Could you check a few things on this model? Use its own coordinates, in mm. Round coordinates to 2 decimals unless told otherwise and drop trailing zeros. Order: outer loops, then holes, each group sorted by start corner. A loop starts at its lowest first (then second) coordinate and runs counter-clockwise, first axis right, second up.
```python
from build123d import *

# Parameters (mm, degrees)
ESBO_O1_R                = 3
RESSALTO_EXTRUS_O1_DEPTH = 36
CHANFRO1_SIZE            = 0.25
ESBO_O2_R                = 2
CORTE_EXTRUS_O1_DEPTH    = 16


with BuildPart() as part:
    # Esboço1 → Ressalto-extrusão1 (new, symmetric)
    with BuildSketch(Plane.XY):
        Circle(ESBO_O1_R)
    extrude(amount=RESSALTO_EXTRUS_O1_DEPTH, both=True)

    # Chanfro1
    chanfro1_edges = [part.edges().sort_by_distance(p)[0] for p in [
        (-3, 0, -36),
        (-3, 0, 36),
    ]]
    chamfer(chanfro1_edges, length=CHANFRO1_SIZE)

    # Esboço2 → Corte-extrusão1 (cut)
    with BuildSketch(Plane.XY.offset(36)):
        Circle(ESBO_O2_R)
    corte_extrus_o1 = extrude(amount=-CORTE_EXTRUS_O1_DEPTH, mode=Mode.SUBTRACT)

    # Espelhar1: Corte-extrusão1 across plane
    add(corte_extrus_o1.mirror(Plane.XY), mode=Mode.SUBTRACT)


solid = part.part
```
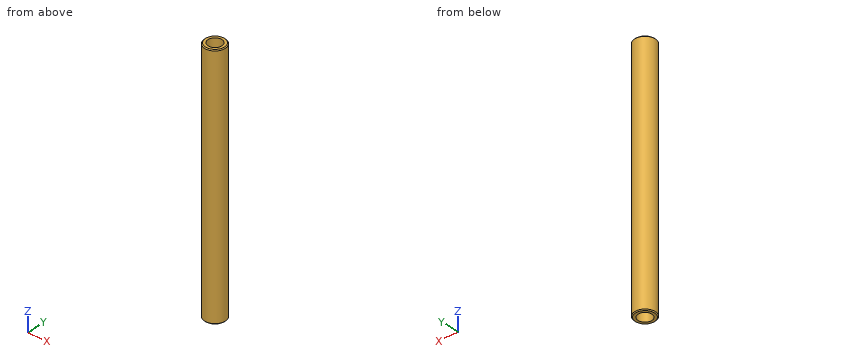
Q1. Imagine slicing it at D-D, the plane z = -6. Please give me the cut outline in (x, y), then the cut area to 3 significant figures.
Q2. For P1, Ø1, axis at x = -2.5, z = 12.5, coming from the -Y side; P2, Ø3, axis at x = 0, y = 0, coming from the -Z side; P3, Ø2.5, axis at x = 0, y = 0, coming from the +Z side, each with a flat end and sliding along its axis, tell me the tip position at first contact or that it passes through.
Q3. Imagine slicing it at B-B, the plane z = 30. Please give me the cut outline in (x, y).
Q4. I need wall thicknesses on L1, parallel to Y at x = 0, z = 25; L2, parallel to Z at x = -0.65, y = 0; L3, parallel to Y at x = 0.65, z = -32. Which ranges of each line are inside material? Lowest first, please.
Q5. Imagine slicing it at A-A, the plane x = 0. Please give me the cut outline in (y, z), then the cut area to 3 significant figures.
Filled in:
1. outline: circle Ø6 at (0, 0)
1. area: 28.3 mm2
2. P1: stops at y = -2.24
2. P2: stops at z = -20
2. P3: stops at z = 20
3. outline: circle Ø6 at (0, 0); hole circle Ø4 at (0, 0)
4. L1: y = -3 to -2, 2 to 3
4. L2: z = -20 to 20
4. L3: y = -2.93 to -1.89, 1.89 to 2.93
5. outline: (-3, -35.75) - (-2.75, -36) - (-2, -36) - (-2, -20) - (2, -20) - (2, -36) - (2.75, -36) - (3, -35.75) - (3, 35.75) - (2.75, 36) - (2, 36) - (2, 20) - (-2, 20) - (-2, 36) - (-2.75, 36) - (-3, 35.75) - close
5. area: 304 mm2
